from build123d import *

# Parameters (mm, degrees)
BOSS_EXTRUDE1_DEPTH = 20
FILLET1_R           = 2.5
SKETCH2_R           = 2.5
CUT_EXTRUDE1_DEPTH  = 21
CHAMFER1_SIZE       = 1


with BuildPart() as part:
    # Sketch1 → Boss-Extrude1 (new body)
    with BuildSketch(Plane(origin=(0, 0, 0), x_dir=(1, 0, 0), z_dir=(0, 1, 0))):
        Polygon((0, 25), (-135, 25), (-135, 40), (15, 40), (15, -40), (-135, -40), (-135, -25), (0, -25), align=None)
    extrude(amount=BOSS_EXTRUDE1_DEPTH)

    # Fillet1
    fillet1_edges = [part.edges().sort_by_distance(p)[0] for p in [
        (-135, 10, -40),
        (15, 10, -40),
        (15, 10, 40),
        (-135, 10, 40),
        (-60, 20, 40),
        (15, 20, 0),
        (-60, 20, -40),
        (-60, 0, -40),
        (15, 0, 0),
        (-60, 0, 40),
    ]]
    fillet(fillet1_edges, radius=FILLET1_R)

    # Sketch2 → Cut-Extrude1 (cut, through all)
    with BuildSketch(Plane(origin=(0, 20, 0), x_dir=(1, 0, 0), z_dir=(0, 1, 0))):
        with Locations((7.5, 32.5)):
            Circle(SKETCH2_R)
        with Locations((7.5, -32.5)):
            Circle(SKETCH2_R)
        with Locations((-127.5, 32.5)):
            Circle(SKETCH2_R)
        with Locations((-127.5, -32.5)):
            Circle(SKETCH2_R)
    extrude(amount=-CUT_EXTRUDE1_DEPTH, mode=Mode.SUBTRACT)

    # Chamfer1
    chamfer1_edges = [part.edges().sort_by_distance(p)[0] for p in [
        (5, 20, 32.5),
        (-130, 20, -32.5),
        (-130, 20, 32.5),
        (5, 20, -32.5),
    ]]
    chamfer(chamfer1_edges, length=CHAMFER1_SIZE)


solid = part.part
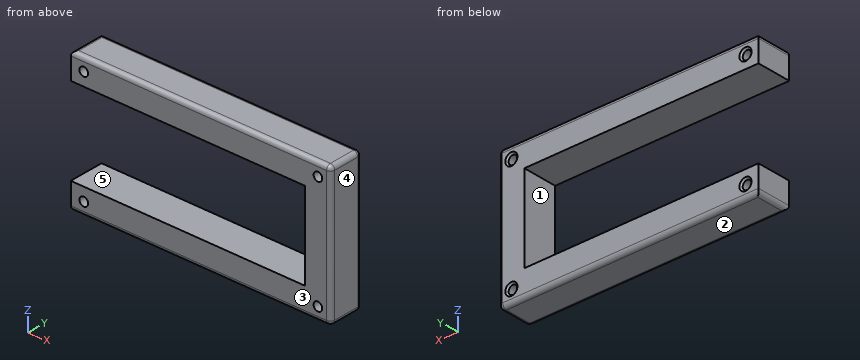
Here's how the part is built. I have some questions about the finished solid (model axes, mm). Face numbers are marked on the shaded views. A direction names the side the tool comes from. Give positions to 0.01 mm unless a question says otherwise; leave off trailing zeros. Order: outer loops, then holes, each group sorted by start corner. A loop starts at its lowest first (then second) coordinate and runs counter-clockwise, first axis right, second up. Notation, with made-up numbers: M 33,-13 L 56,-13 A29 ccw 56,9 Z; hole C -36,46 d6. An arc over 180 degrees is marked long. Answer as a JSON object with one key per item and string values. Group by question number.
1) On a 3-axis mill with a long thin cutter (end or side, diameter ignored), from which of +Z, -Z, +X, -X, +Y, -Y can I reach the whole of each face in a straight line? I mean the marked faces 4 and 5. Say none if no direction works.
2) Please list where these lines run through material, in increasing order: L1, parallel to Z at x = -127.5, y = 12.25; L2, parallel to X at y = 6.75, z = -32.5; L3, parallel to Z at x = -24, y = 8.5. Write a range as [from, to].
3) Suppose I cut it at B-B, the plane z = -32.5. Write out the boundary of the cut face in (x, y).
4) Suppose I cut it at D-D, the plane y = 8.5. Write out the boundary of the cut face in (x, z), plus the area to 3 significant figures.
5) We'd pull the mould along Z, two halves only. Please class the marked faces 1, 2 and 3: pulls with the +Z half, pulls with the -Z half, needs draft (parallel to the pull), parting line crosses it, or undercut.
6) I'm going to push flat-ended pins straight in: pin 1 Ø3 at (x, z) = (-127.5, 32.5) entering from -Y; pin 2 Ø6 at (x, z) = (-127.5, -32.5) entering from +Y. Where does each tip first touch, or does it pass through?
7) Suppose I cut it at A-A, the plane x = -127.5. Write out the boundary of the cut face in (y, z).
8) Suppose I cut it at C-C, the plane x = 7.5. Write out the boundary of the cut face in (y, z).
Results found:
{
 "1": {"face 4": "+Z, -Z, +X, +Y, -Y", "face 5": "-X, +Y, -Y"},
 "2": {"L1": "[-40, -35], [-30, -25], [25, 30], [35, 40]", "L2": "[-135, -130], [-125, 5], [10, 15]", "L3": "[-40, -25], [25, 40]"},
 "3": {"outline": "M -135,0 L -130,0 L -130,19 L -131,20 L -135,20 Z; M -125,0 L 5,0 L 5,19 L 4,20 L -124,20 L -125,19 Z; M 10,0 L 12.5,0 A2.5 ccw 15,2.5 L 15,17.5 A2.5 ccw 12.5,20 L 11,20 L 10,19 Z"},
 "4": {"outline": "M -135,-37.5 A2.5 ccw -132.5,-40 L 12.5,-40 A2.5 ccw 15,-37.5 L 15,37.5 A2.5 ccw 12.5,40 L -132.5,40 A2.5 ccw -135,37.5 L -135,25 L 0,25 L 0,-25 L -135,-25 Z; hole C -127.5,-32.5 d5; hole C -127.5,32.5 d5; hole C 7.5,-32.5 d5; hole C 7.5,32.5 d5", "area": "5,170 mm²"},
 "5": {"face 1": "undercut", "face 2": "pulls with the -Z half", "face 3": "needs draft"},
 "6": {"pin 1": "through", "pin 2": "y = 19.5"},
 "7": {"outline": "M 0,-37.5 A2.5 ccw 2.5,-40 L 17.5,-40 A2.5 ccw 20,-37.5 L 20,-36 L 19,-35 L 0,-35 Z; M 0,-30 L 19,-30 L 20,-29 L 20,-25 L 0,-25 Z; M 0,25 L 20,25 L 20,29 L 19,30 L 0,30 Z; M 0,35 L 19,35 L 20,36 L 20,37.5 A2.5 ccw 17.5,40 L 2.5,40 A2.5 ccw 0,37.5 Z"},
 "8": {"outline": "M 0,-37.5 A2.5 ccw 2.5,-40 L 17.5,-40 A2.5 ccw 20,-37.5 L 20,-36 L 19,-35 L 0,-35 Z; M 0,-30 L 19,-30 L 20,-29 L 20,29 L 19,30 L 0,30 Z; M 0,35 L 19,35 L 20,36 L 20,37.5 A2.5 ccw 17.5,40 L 2.5,40 A2.5 ccw 0,37.5 Z"}
}
